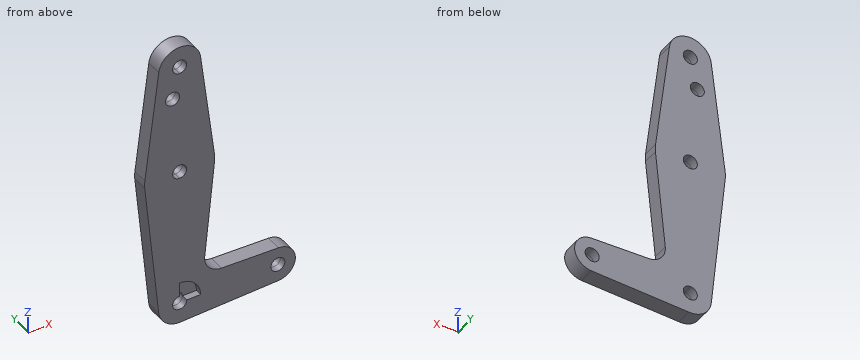
```python
from build123d import *

# Parameters (mm, degrees)
F0_R     = 3.175
F1_DEPTH = 4.064
F2_DEPTH = 3.048


with BuildPart() as f1:
    # F0 (on Front) → F1 (new body)
    with BuildSketch(Plane.XZ):
        with BuildLine():
            ThreePointArc((15.7954255641, -1.5875), (15.8550939106, -0.7947465541), (15.875, 0))
            ThreePointArc((15.875, 0), (15.8438414904, 0.9941387366), (15.7504882737, 1.984375))
            ThreePointArc((15.7504882737, 1.984375), (10.5003255158, 11.90625), (0, 15.875))
            Line((0, 15.875), (0, 3.175))
            ThreePointArc((0, 3.175), (2.2450640303, 2.2450640303), (3.175, 0))
            ThreePointArc((3.175, 0), (2.2450640303, -2.2450640303), (0, -3.175))
            Line((0, -3.175), (0, -15.875))
            ThreePointArc((0, -15.875), (10.6492737428, -11.7732150983), (15.7954255641, -1.5875))
        make_face()
        with BuildLine():
            ThreePointArc((0, 15.875), (10.5003255158, 11.90625), (15.7504882737, 1.984375))
            Line((15.7504882737, 1.984375), (9.4502929642, 51.990625))
            ThreePointArc((9.4502929642, 51.990625), (9.5063048942, 51.396483242), (9.525, 50.8))
            ThreePointArc((9.525, 50.8), (6.7351920908, 44.0648079092), (0, 41.275))
            Line((0, 41.275), (0, 36.5252))
            Line((0, 36.5252), (0, 29.7381002456))
            Line((0, 29.7381002456), (0, 15.875))
        make_face()
        with BuildLine():
            Line((11.3411865923, -45.9066181876), (15.7954255641, -1.5875))
            ThreePointArc((15.7954255641, -1.5875), (10.6492737428, -11.7732150983), (0, -15.875))
            Line((0, -15.875), (0, -53.975))
            ThreePointArc((0, -53.975), (6.7351920908, -56.7648079092), (9.525, -63.5))
            Line((9.525, -63.5), (36.5125, -63.5))
            ThreePointArc((36.5125, -63.5), (38.9384772185, -57.7879930953), (44.7334821429, -55.5675637964))
            Line((44.7334821429, -55.5675637964), (18.9676000005, -54.6467662892))
            ThreePointArc((18.9676000005, -54.6467662892), (13.2611998974, -51.9286408502), (11.3411865923, -45.9066181876))
        make_face()
        with BuildLine():
            Line((0, 3.175), (0, 15.875))
            ThreePointArc((0, 15.875), (-10.5003255158, 11.90625), (-15.7504882737, 1.984375))
            ThreePointArc((-15.7504882737, 1.984375), (-15.8737438155, 0.1997054867), (-15.7954255641, -1.5875))
            ThreePointArc((-15.7954255641, -1.5875), (-10.6492737428, -11.7732150983), (0, -15.875))
            Line((0, -15.875), (0, -3.175))
            ThreePointArc((0, -3.175), (-3.175, 0), (0, 3.175))
        make_face()
        with BuildLine():
            ThreePointArc((-15.7504882737, 1.984375), (-10.5003255158, 11.90625), (0, 15.875))
            Line((0, 15.875), (0, 29.7381002456))
            Line((0, 29.7381002456), (0, 36.5252))
            Line((0, 36.5252), (0, 41.275))
            ThreePointArc((0, 41.275), (-7.14375, 44.4998046905), (-9.4502929642, 51.990625))
            Line((-9.4502929642, 51.990625), (-15.7504882737, 1.984375))
        make_face()
        with Locations((-3.175, 36.5252)):
            Circle(F0_R, mode=Mode.SUBTRACT)
        with BuildLine():
            ThreePointArc((9.525, 50.8), (9.5063048942, 51.396483242), (9.4502929642, 51.990625))
            ThreePointArc((9.4502929642, 51.990625), (0, 60.325), (-9.4502929642, 51.990625))
            ThreePointArc((-9.4502929642, 51.990625), (-7.14375, 44.4998046905), (0, 41.275))
            ThreePointArc((0, 41.275), (6.7351920908, 44.0648079092), (9.525, 50.8))
        make_face()
        with BuildLine():
            ThreePointArc((3.175, 50.8), (2.2450640303, 48.5549359697), (0, 47.625))
            ThreePointArc((0, 47.625), (-2.2450640303, 53.0450640303), (3.175, 50.8))
        make_face(mode=Mode.SUBTRACT)
        with BuildLine():
            Line((0, -53.975), (0, -15.875))
            ThreePointArc((0, -15.875), (-10.6492737428, -11.7732150983), (-15.7954255641, -1.5875))
            Line((-15.7954255641, -1.5875), (-9.4772553384, -64.4525))
            ThreePointArc((-9.4772553384, -64.4525), (-7.063929059, -57.1104357543), (0, -53.975))
        make_face()
        with BuildLine():
            Line((0, -60.325), (0, -53.975))
            ThreePointArc((0, -53.975), (-7.063929059, -57.1104357543), (-9.4772553384, -64.4525))
            ThreePointArc((-9.4772553384, -64.4525), (-6.3895642457, -70.563929059), (0, -73.025))
            Line((0, -73.025), (0.6773435479, -73.000885786))
            ThreePointArc((0.6773435479, -73.000885786), (6.9705567315, -69.9912990883), (9.525, -63.5))
            Line((9.525, -63.5), (3.175, -63.5))
            ThreePointArc((3.175, -63.5), (-2.2450640303, -65.7450640303), (0, -60.325))
        make_face()
        with BuildLine():
            Line((36.5125, -63.5), (9.525, -63.5))
            ThreePointArc((9.525, -63.5), (6.9705567315, -69.9912990883), (0.6773435479, -73.000885786))
            Line((0.6773435479, -73.000885786), (44.7324052746, -71.4324746146))
            ThreePointArc((44.7324052746, -71.4324746146), (38.9380895153, -69.2116327839), (36.5125, -63.5))
        make_face()
        with BuildLine():
            ThreePointArc((52.3875, -63.5), (50.1620069047, -57.9884772185), (44.7334821429, -55.5675637964))
            ThreePointArc((44.7334821429, -55.5675637964), (38.9384772185, -57.7879930953), (36.5125, -63.5))
            ThreePointArc((36.5125, -63.5), (38.9380895153, -69.2116327839), (44.7324052746, -71.4324746146))
            ThreePointArc((44.7324052746, -71.4324746146), (50.1616327839, -69.0119104847), (52.3875, -63.5))
        make_face()
        with BuildLine():
            ThreePointArc((47.625, -63.5), (44.45, -66.675), (41.275, -63.5))
            ThreePointArc((41.275, -63.5), (44.45, -60.325), (47.625, -63.5))
        make_face(mode=Mode.SUBTRACT)
        with BuildLine():
            Line((0.6773435479, -73.000885786), (0, -73.025))
            ThreePointArc((0, -73.025), (0.3388863295, -73.0189695375), (0.6773435479, -73.000885786))
        make_face()
        with BuildLine():
            ThreePointArc((9.525, -63.5), (6.7351920908, -56.7648079092), (0, -53.975))
            Line((0, -53.975), (0, -60.325))
            ThreePointArc((0, -60.325), (2.2450640303, -61.2549359697), (3.175, -63.5))
            Line((3.175, -63.5), (9.525, -63.5))
        make_face()
    extrude(amount=-F1_DEPTH)

    # F0 (on Front) → F2 (join)
    with BuildSketch(Plane.XZ):
        with BuildLine():
            ThreePointArc((15.7954255641, -1.5875), (15.8550939106, -0.7947465541), (15.875, 0))
            ThreePointArc((15.875, 0), (15.8438414904, 0.9941387366), (15.7504882737, 1.984375))
            ThreePointArc((15.7504882737, 1.984375), (10.5003255158, 11.90625), (0, 15.875))
            Line((0, 15.875), (0, 3.175))
            ThreePointArc((0, 3.175), (2.2450640303, 2.2450640303), (3.175, 0))
            ThreePointArc((3.175, 0), (2.2450640303, -2.2450640303), (0, -3.175))
            Line((0, -3.175), (0, -15.875))
            ThreePointArc((0, -15.875), (10.6492737428, -11.7732150983), (15.7954255641, -1.5875))
        make_face()
        with BuildLine():
            ThreePointArc((0, 15.875), (10.5003255158, 11.90625), (15.7504882737, 1.984375))
            Line((15.7504882737, 1.984375), (9.4502929642, 51.990625))
            ThreePointArc((9.4502929642, 51.990625), (9.5063048942, 51.396483242), (9.525, 50.8))
            ThreePointArc((9.525, 50.8), (6.7351920908, 44.0648079092), (0, 41.275))
            Line((0, 41.275), (0, 36.5252))
            Line((0, 36.5252), (0, 29.7381002456))
            Line((0, 29.7381002456), (0, 15.875))
        make_face()
        with BuildLine():
            Line((11.3411865923, -45.9066181876), (15.7954255641, -1.5875))
            ThreePointArc((15.7954255641, -1.5875), (10.6492737428, -11.7732150983), (0, -15.875))
            Line((0, -15.875), (0, -53.975))
            ThreePointArc((0, -53.975), (6.7351920908, -56.7648079092), (9.525, -63.5))
            Line((9.525, -63.5), (36.5125, -63.5))
            ThreePointArc((36.5125, -63.5), (38.9384772185, -57.7879930953), (44.7334821429, -55.5675637964))
            Line((44.7334821429, -55.5675637964), (18.9676000005, -54.6467662892))
            ThreePointArc((18.9676000005, -54.6467662892), (13.2611998974, -51.9286408502), (11.3411865923, -45.9066181876))
        make_face()
        with BuildLine():
            Line((0, 3.175), (0, 15.875))
            ThreePointArc((0, 15.875), (-10.5003255158, 11.90625), (-15.7504882737, 1.984375))
            ThreePointArc((-15.7504882737, 1.984375), (-15.8737438155, 0.1997054867), (-15.7954255641, -1.5875))
            ThreePointArc((-15.7954255641, -1.5875), (-10.6492737428, -11.7732150983), (0, -15.875))
            Line((0, -15.875), (0, -3.175))
            ThreePointArc((0, -3.175), (-3.175, 0), (0, 3.175))
        make_face()
        with BuildLine():
            ThreePointArc((-15.7504882737, 1.984375), (-10.5003255158, 11.90625), (0, 15.875))
            Line((0, 15.875), (0, 29.7381002456))
            Line((0, 29.7381002456), (0, 36.5252))
            Line((0, 36.5252), (0, 41.275))
            ThreePointArc((0, 41.275), (-7.14375, 44.4998046905), (-9.4502929642, 51.990625))
            Line((-9.4502929642, 51.990625), (-15.7504882737, 1.984375))
        make_face()
        with Locations((-3.175, 36.5252)):
            Circle(F0_R, mode=Mode.SUBTRACT)
        with BuildLine():
            ThreePointArc((9.525, 50.8), (9.5063048942, 51.396483242), (9.4502929642, 51.990625))
            ThreePointArc((9.4502929642, 51.990625), (0, 60.325), (-9.4502929642, 51.990625))
            ThreePointArc((-9.4502929642, 51.990625), (-7.14375, 44.4998046905), (0, 41.275))
            ThreePointArc((0, 41.275), (6.7351920908, 44.0648079092), (9.525, 50.8))
        make_face()
        with BuildLine():
            ThreePointArc((3.175, 50.8), (2.2450640303, 48.5549359697), (0, 47.625))
            ThreePointArc((0, 47.625), (-2.2450640303, 53.0450640303), (3.175, 50.8))
        make_face(mode=Mode.SUBTRACT)
        with BuildLine():
            Line((0, -53.975), (0, -15.875))
            ThreePointArc((0, -15.875), (-10.6492737428, -11.7732150983), (-15.7954255641, -1.5875))
            Line((-15.7954255641, -1.5875), (-9.4772553384, -64.4525))
            ThreePointArc((-9.4772553384, -64.4525), (-7.063929059, -57.1104357543), (0, -53.975))
        make_face()
        with BuildLine():
            Line((0, -60.325), (0, -53.975))
            ThreePointArc((0, -53.975), (-7.063929059, -57.1104357543), (-9.4772553384, -64.4525))
            ThreePointArc((-9.4772553384, -64.4525), (-6.3895642457, -70.563929059), (0, -73.025))
            Line((0, -73.025), (0.6773435479, -73.000885786))
            ThreePointArc((0.6773435479, -73.000885786), (6.9705567315, -69.9912990883), (9.525, -63.5))
            Line((9.525, -63.5), (3.175, -63.5))
            ThreePointArc((3.175, -63.5), (-2.2450640303, -65.7450640303), (0, -60.325))
        make_face()
        with BuildLine():
            Line((36.5125, -63.5), (9.525, -63.5))
            ThreePointArc((9.525, -63.5), (6.9705567315, -69.9912990883), (0.6773435479, -73.000885786))
            Line((0.6773435479, -73.000885786), (44.7324052746, -71.4324746146))
            ThreePointArc((44.7324052746, -71.4324746146), (38.9380895153, -69.2116327839), (36.5125, -63.5))
        make_face()
        with BuildLine():
            ThreePointArc((52.3875, -63.5), (50.1620069047, -57.9884772185), (44.7334821429, -55.5675637964))
            ThreePointArc((44.7334821429, -55.5675637964), (38.9384772185, -57.7879930953), (36.5125, -63.5))
            ThreePointArc((36.5125, -63.5), (38.9380895153, -69.2116327839), (44.7324052746, -71.4324746146))
            ThreePointArc((44.7324052746, -71.4324746146), (50.1616327839, -69.0119104847), (52.3875, -63.5))
        make_face()
        with BuildLine():
            ThreePointArc((47.625, -63.5), (44.45, -66.675), (41.275, -63.5))
            ThreePointArc((41.275, -63.5), (44.45, -60.325), (47.625, -63.5))
        make_face(mode=Mode.SUBTRACT)
        with BuildLine():
            Line((0.6773435479, -73.000885786), (0, -73.025))
            ThreePointArc((0, -73.025), (0.3388863295, -73.0189695375), (0.6773435479, -73.000885786))
        make_face()
    extrude(amount=F2_DEPTH)


solid = f1.part
```
Read the model definition and answer for the solid it produces. Units are mm, in the model's axes. Give positions to 0.01 mm unless a question says otherwise; leave off trailing zeros. Order: outer loops, then holes, each group sorted by start corner. A loop starts at its lowest first (then second) coordinate and runs counter-clockwise, first axis right, second up. Notation, with made-up numbers: (53, -29.5) -> (89, -29.5) arc R23 ccw to (89, 0.5) -> close; hole circle Ø5 at (44.25, 77.25). An arc over 180 degrees is marked (long way). One line per item, written item: value. Start each with the question number.
(1) The part is cut by section B-B (x = 7). Determine the outline of the cut face in (y, z), and give its area (3 significant figures).
(2) Straight lines are drawn through the part: L1, parallel to Z at x = 44.45, y = 0.9 (3 decimals); L2, parallel to Z at x = -1.5, y = -1.5; L3, parallel to Z at x = 42, y = 1.25. For each, find the intervals that lie inside material, in ascending order.
(3) The part is cut by section C-C (z = -18). Determine the outline of the cut face in (x, y), and give its area (3 significant figures).
(4) The part is cut by section A-A (y = -1.75). State how many separate pieces and enclosed holes the cut face has, and give its area (3 significant figures).
(5) Flat-ended cylindrical pins translate along their axes: P1, Ø3, axis at y = -1.5, z = -10.5, coming from the -X side; P2, Ø4, axis at y = 1, z = -49, coming from the +X side; P3, Ø8.5, axis at x = 0, z = 50.8, coming from the -Y side; P4, Ø1.5, axis at y = -1, z = -57.5, coming from the +X side. Find the tip coordinate at first contact, or state that the pin passes through.
(6) The part is cut by section D-D (x = 31.5). Determine the outline of the cut face in (y, z).
Taken from the geometry:
1. outline: (-3.05, -72.78) -> (4.06, -72.78) -> (4.06, 57.26) -> (-3.05, 57.26) -> (-3.05, -57.04) -> (0, -57.04) -> (0, -63.5) -> (-3.05, -63.5) -> close
1. area: 905 mm^2
2. L1: -71.443 to -66.675, -60.325 to -55.557
2. L2: -72.91 to -66.3, -60.7 to -2.8, 2.8 to 33.83, 39.22 to 48, 53.6 to 60.21
2. L3: -71.53 to -65.52, -61.48 to -55.47
3. outline: (-14.15, -3.05) -> (14.15, -3.05) -> (14.15, 4.06) -> (-14.15, 4.06) -> close
3. area: 201 mm^2
4. separate pieces: 1
4. enclosed holes: 5
4. area: 3,710 mm^2
5. P1: x = -15.05
5. P2: x = 12.56
5. P3: y = -3.05
5. P4: x = 50.4
6. outline: (-3.05, -71.9) -> (4.06, -71.9) -> (4.06, -55.09) -> (-3.05, -55.09) -> close
